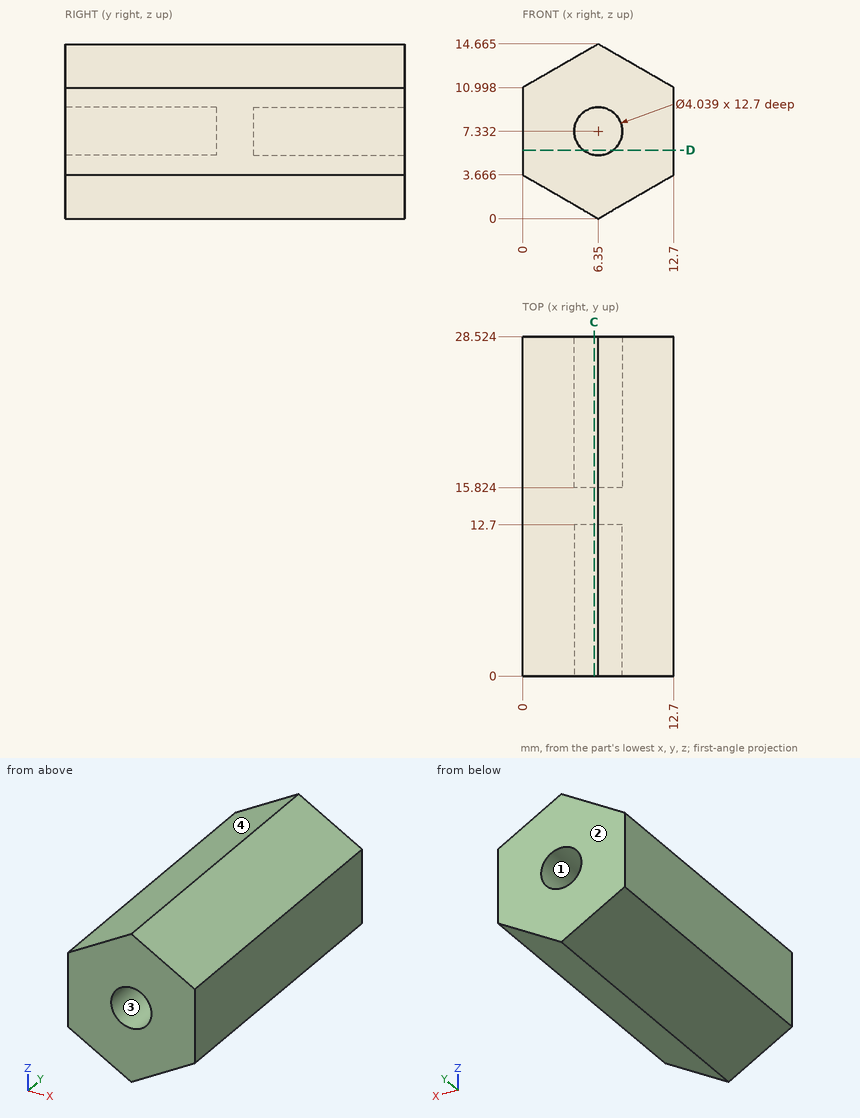
The drawing under review shows one solid part. Ordinate dimensions are in mm from its lowest x, y, z. Round coordinates to 2 decimals unless told otherwise and drop trailing zeros. Write each loop counter-clockwise with the first axis right and the second up, starting at its lowest first coordinate (ties: lowest second). Pieces come first, ordered by that corner, then holes.
(1) We need section D-D on z = 5.75. Give the boundary of the cut face in (x, y) (1 decimal).
(2) Insertion check: pin 1 (2 mm diameter, centred on x = 7, y = 4.5, fed in from +Z) (1 decimal); pin 2 (2 mm diameter, centred on x = 9.5, y = 5, fed in from -Z); pin 3 (4 mm diameter, centred on x = 11.5, y = 13.5, fed in from +Z) (1 decimal); pin 4 (3 mm diameter, centred on x = 6, z = 7.5, fed in from -Y). Each pin has a flat end and moves straight along its axis. Give the tip position at first contact, or say it passes through.
(3) We need section C-C on x = 6. Give the boundary of the cut face in (y, z) (1 decimal), and give its area (3 significant figures).
(4) Wall thickness on L1, parallel to X at y = 6, z = 7.5; L2, parallel to X at y = 1.5, z = 8.5 (1 decimal); L3, parallel to Z at x = 9.75, y = 18.25 (1 decimal): over which ranges is each line inside the solid? List them lowest first.
(5) Mouldability with a two-part tool opening along Z and no side actions: class the marked faces 1, 2, 3 and 4 as +Z half, -Z half, draft (parallel to the pull), parting line (faces both ways), or undercut.
Findings below:
1. outline: (0, 0) - (5.1, 0) - (5.1, 12.7) - (7.6, 12.7) - (7.6, 0) - (12.7, 0) - (12.7, 28.5) - (7.6, 28.5) - (7.6, 15.8) - (5.1, 15.8) - (5.1, 28.5) - (0, 28.5) - close
2. pin 1: stops at z = 14.7
2. pin 2: stops at z = 1.24
2. pin 3: stops at z = 12.8
2. pin 4: stops at y = 12.7
3. outline: (0, 0.2) - (28.5, 0.2) - (28.5, 5.3) - (15.8, 5.3) - (15.8, 9.3) - (28.5, 9.3) - (28.5, 14.5) - (0, 14.5) - (0, 9.3) - (12.7, 9.3) - (12.7, 5.3) - (0, 5.3) - close
3. area: 306 mm2
4. L1: x = 0 to 4.34, 8.36 to 12.7
4. L2: x = 0 to 4.7, 8 to 12.7
4. L3: z = 2 to 12.7
5. face 1: undercut
5. face 2: draft
5. face 3: undercut
5. face 4: +Z half
